Geometry: final body of the model. Coordinates: model frame, mm. Face numbers are marked on the shaded views. Coordinates: 2 decimals unless noted, no trailing zeros. Loops run counter-clockwise (first coordinate to the right, second up) from the corner with the lowest first, then second, coordinate; pieces in that order, holes last. Notation, with made-up numbers: (-18, -9.5) - (37, -9.5) arc R7 cw to (37, -0.5) - close; hole circle Ø8 at (-10, 32). An arc over 180 degrees is marked (long way). Answer in a Markdown table with one row per item.
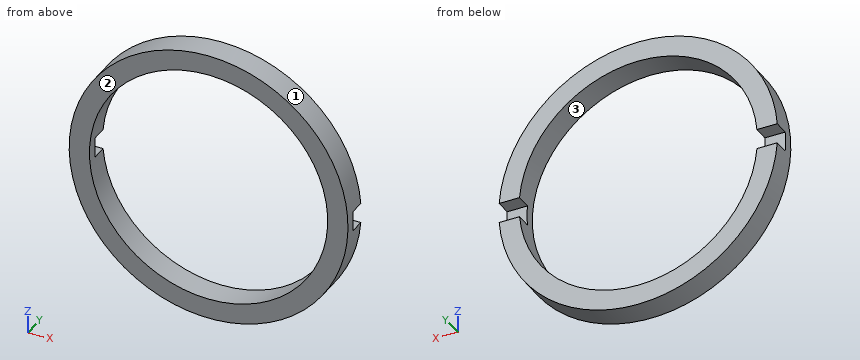
from build123d import *

# Parameters (mm, degrees)
SKETCH_1_W          = 2
SKETCH_1_H          = 2.5
SKETCH_2_W          = 53.705080546
SKETCH_2_H          = 2
CUT_EXTRUDE_1_DEPTH = 1.5


with BuildPart() as part:
    # 草图1 → 旋转1 (revolve)
    with BuildSketch(Plane.XY, mode=Mode.PRIVATE) as revolve_1_sk:
        with Locations((12.75, -3.214249787)):
            Rectangle(SKETCH_1_W, SKETCH_1_H)
    revolve(revolve_1_sk.sketch.rotate(Axis((0, 56.260842627, 0), (0, -1, 0)), 90), axis=Axis((0, 56.260842627, 0), (0, -1, 0)))  # turned: the seam where the file's is

    # 草图2 → 切除-拉伸1 (cut)
    with BuildSketch(Plane(origin=(0, -1.964249787, 0), x_dir=(1, 0, 0), z_dir=(0, 1, 0))):
        Rectangle(SKETCH_2_W, SKETCH_2_H)
    extrude(amount=-CUT_EXTRUDE_1_DEPTH, mode=Mode.SUBTRACT)


solid = part.part
(1) Cut plane A-A on z = 0. Output: boundary loops of the cut face in (x, y).
Verdict:
| item | result |
|---|---|
| outline | (-13.75, -4.46) - (-11.75, -4.46) - (-11.75, -3.46) - (-13.75, -3.46) - close; (11.75, -4.46) - (13.75, -4.46) - (13.75, -3.46) - (11.75, -3.46) - close |
(2) Pull-direction query (Z, two-part tool) for the marked faces 1, 2 and 3; classes: pulls with the +Z half, pulls with the -Z half, needs draft (parallel to the pull), parting line crosses it, or undercut.
Verdict:
| item | result |
|---|---|
| face 1 | parting line crosses it |
| face 2 | needs draft |
| face 3 | undercut |
(3) First-contact query: pin 1 Ø0.8 at (x, y) = (13, -2.5) entering from -Z; pin 2 Ø0.8 at (x, y) = (-13, -2.5) entering from +Z. Flat tips, straight axial feed; report the tip coordinate or a pass-through.
Verdict:
| item | result |
|---|---|
| pin 1 | stops at z = -5.5 |
| pin 2 | stops at z = 5.5 |
(4) Ray query, probe 1 along X at (y, z) = (-3.8, 0); probe 2 along Z at (x, y) = (10.75, -3.4); probe 3 along X at (y, z) = (-2.55, -8.25). Return the intervals inside material, ascending.
Verdict:
| item | result |
|---|---|
| probe 1 | x = -13.75 to -11.75, 11.75 to 13.75 |
| probe 2 | z = -8.57 to -4.74, 4.74 to 8.57 |
| probe 3 | x = -11 to -8.37, 8.37 to 11 |
